The figure shows three views and two pictorial views of one solid part (mm, origin at its lowest corner). Answer the questions. Coordinates: 2 decimals unless noted, no trailing zeros. Write each loop counter-clockwise with the first axis right and the second up, starting at its lowest first coordinate (ties: lowest second). Pieces come first, ordered by that corner, then holes.
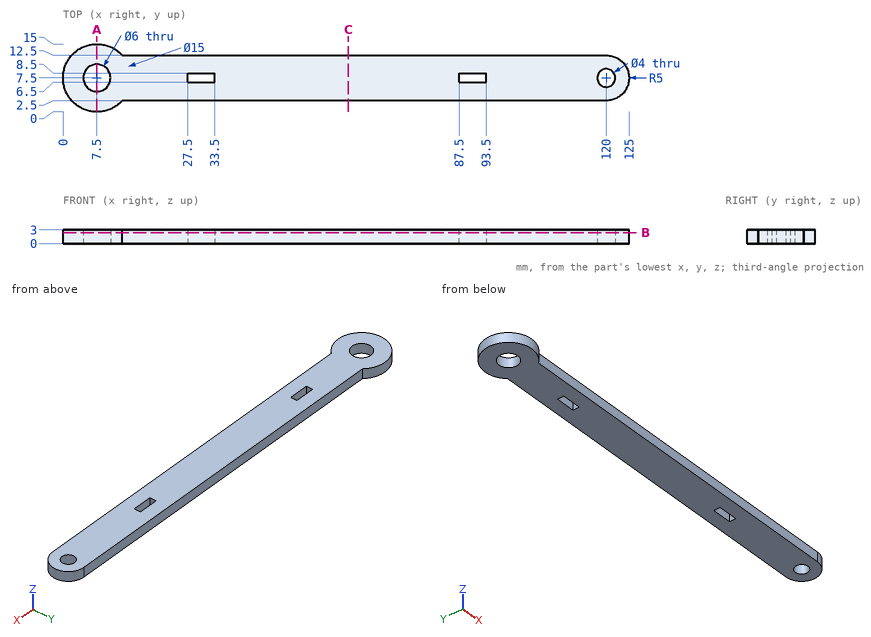
Q1. The part is cut by section A-A, the plane x = 7.5. Write down the section's boundary in (y, z), then the cut area to 3 significant figures.
Answers below:
outline: (0, 0) - (4.5, 0) - (4.5, 3) - (0, 3) - close; (10.5, 0) - (15, 0) - (15, 3) - (10.5, 3) - close
area: 27.0 mm2
Q2. Find the intervals of material crossed by probe 1 along Y at (x, z) = (120, 2.1); probe 2 along Y at (x, z) = (37.5, 2.75); probe 3 along X at (y, z) = (10.25, 0.95), in increasing order.
Answers below:
probe 1: y = 2.5 to 5.5, 9.5 to 12.5
probe 2: y = 2.5 to 12.5
probe 3: x = 0.52 to 6.3, 8.7 to 124.18
Q3. The part is cut by section C-C, the plane x = 63. Write down the section's boundary in (y, z).
Answers below:
outline: (2.5, 0) - (12.5, 0) - (12.5, 3) - (2.5, 3) - close
Q4. The part is cut by section B-B, the plane z = 2.4. Write down the section's boundary in (x, y).
Answers below:
outline: (13.09, 2.5) - (120, 2.5) arc R5 ccw to (120, 12.5) - (13.09, 12.5) arc R7.5 ccw (long way) to start; hole circle Ø6 at (7.5, 7.5); hole (27.5, 6.5) - (33.5, 6.5) - (33.5, 8.5) - (27.5, 8.5) - close; hole (87.5, 6.5) - (93.5, 6.5) - (93.5, 8.5) - (87.5, 8.5) - close; hole circle Ø4 at (120, 7.5)
Q5. Given pin 1 (0.9 mm diameter, centred on x = 90.5, z = 1.5, fed in from +Y); pin 2 (1.6 mm diameter, centred on y = 7, z = 1, fed in from +X); pin 3 (1 mm diameter, centred on y = 12.5, z = 0.5, fed in from -X); pin 4 (1 mm diameter, centred on x = 50.5, z = 0.5, fed in from -Y), each flat-ended and moving along its own axis, determine where each tip first touches the part or whether it passes through.
Answers below:
pin 1: stops at y = 12.5
pin 2: stops at x = 125
pin 3: stops at x = 1.5
pin 4: stops at y = 2.5
